Here's how the part is built. I have some questions about the finished solid (model axes, mm). Give positions to 0.01 mm unless a question says otherwise; leave off trailing zeros. Write each loop counter-clockwise with the first axis right and the second up, starting at its lowest first coordinate (ties: lowest second). Pieces come first, ordered by that corner, then holes. Notation, with made-up numbers: (68, -4.5) -> (97, -4.5) arc R16 cw to (97, 15.5) -> close; hole circle Ø4 at (85, 34). An arc over 180 degrees is marked (long way). Use CSV: the item, a comma, the result in double quotes. Start each with the question number.
(1) For pin 1 Ø6 at (x, z) = (1, 160.5) entering from -Y; pin 2 Ø1 at (y, z) = (-2, 67.5) entering from -X; pin 3 Ø4 at (x, z) = (-24.5, 28.5) entering from +Y, each with a flat end and sliding along its axis, tell me the tip position at first contact or that it passes through.
(2) I need wall thicknesses on L1, parallel to X at y = -23.5, z = 49; L2, parallel to X at y = -34, z = 229; L3, parallel to Y at x = -14, z = 265. Which ranges of each line are inside material? Lowest first, please. Write a range as [from, to].
(3) Suppose I cut it at C-C on z = 20. List the corners of the cut face in (x, y) for me.
(4) Suppose I cut it at A-A on x = 0. List the corners of the cut face in (y, z) for me, plus the area to 3 significant figures.
(5) Suppose I cut it at B-B on y = 49. List the corners of the cut face in (x, z) for me.
from build123d import *

# Parameters (mm, degrees)
SKETCH2_R               = 64.77
SKETCH2_R_2             = 64.516
BOSS_EXTRUDE1_DEPTH     = 279.4
CUT_EXTRUDE1_REACH      = 316.706
CUT_EXTRUDE1_END_RADIUS = 64.516
SKETCH5_W               = 279.4
SKETCH5_H               = 1.016


with BuildPart() as part:
    # Sketch2 → Boss-Extrude1 (new body)
    with BuildSketch(Plane.XY):
        Circle(SKETCH2_R)
        Circle(SKETCH2_R_2, mode=Mode.SUBTRACT)
    extrude(amount=BOSS_EXTRUDE1_DEPTH)

    # Cut-Extrude1: up to this cylinder (the profile starts outside it)
    cut_extrude1_end = Plane(origin=(0, 0, 139.7), z_dir=(0, 0, -1)) * Cylinder(CUT_EXTRUDE1_END_RADIUS, 763.444, mode=Mode.PRIVATE)
    # Sketch5 → Cut-Extrude1 (cut, up to the surface)
    with BuildSketch(Plane.ZY.offset(64.77), mode=Mode.PRIVATE) as cut_extrude1_sk1:
        with Locations((139.7, 0)):
            Rectangle(SKETCH5_W, SKETCH5_H)
    cut_extrude1_tool1 = extrude(cut_extrude1_sk1.sketch, amount=-CUT_EXTRUDE1_REACH, mode=Mode.PRIVATE) - cut_extrude1_end
    add(cut_extrude1_tool1.solids().sort_by_distance((-64.77, 0, 139.7))[0], mode=Mode.SUBTRACT)


solid = part.part
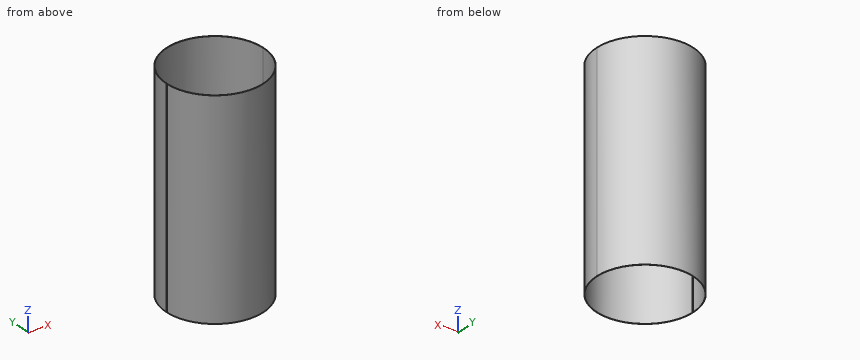
Geometry says:
1,pin 1,"y = -64.77"
1,pin 2,"x = -64.75"
1,pin 3,"y = 60.74"
2,L1,"[-60.36, -60.08], [60.08, 60.36]"
2,L2,"[-55.13, -54.83], [54.83, 55.13]"
2,L3,"[-63.24, -62.98], [62.98, 63.24]"
3,outline,"(-64.77, -0.51) arc R64.77 ccw (long way) to (-64.77, 0.51) -> (-64.51, 0.51) arc R64.52 cw (long way) to (-64.51, -0.51) -> close"
4,outline,"(-64.77, 0) -> (-64.52, 0) -> (-64.52, 279.4) -> (-64.77, 279.4) -> close; (64.52, 0) -> (64.77, 0) -> (64.77, 279.4) -> (64.52, 279.4) -> close"
4,area,"142 mm²"
5,outline,"(-42.36, 0) -> (-41.97, 0) -> (-41.97, 279.4) -> (-42.36, 279.4) -> close; (41.97, 0) -> (42.36, 0) -> (42.36, 279.4) -> (41.97, 279.4) -> close"
